Geometry check sheet. Reference: the model listing, model coordinates, mm. Face numbers are marked on the shaded views. A direction names the side the tool comes from. Give positions to 0.01 mm unless a question says otherwise; leave off trailing zeros. Loops run counter-clockwise (first coordinate to the right, second up) from the corner with the lowest first, then second, coordinate; pieces in that order, holes last.
1. Cross-section at A-A, the plane x = 0. Record the cut outline in (y, z), plus the area to 3 significant figures.
2. Release check for a two-part mould opening along Y. For the marked faces 4, 5 and 6 record: +Y half, -Y half, draft (parallel to the pull), parting line (faces both ways), or undercut.
3. Cross-section at D-D, the plane x = 6.5. Record the cut outline in (y, z), plus the area to 3 significant figures.
4. Cross-section at B-B, the plane z = 0. Record the cut outline in (x, y).
5. Cross-section at C-C, the plane y = -9.25. Record the cut outline in (x, z), plus the area to 3 significant figures.
6. Go/stop test with flat-tipped pins: pin 1 Ø7 at (x, z) = (0, 1.5) entering from +Y; pin 2 Ø8 at (x, y) = (8.5, 0.5) entering from -Z; pin 3 Ø1.5 at (x, y) = (-3.5, -0.5) entering from +Z; pin 4 Ø1.9 at (x, z) = (-1, 0.5) entering from -Y. Record where each tip stops, or that it passes through.
7. Tool access check on the marked faces 1, 2 and 3. Record the directions out of +Z, -Z, +X, -X, +Y, -Y that give a thin tool (end or side, any length) a straight path to the whole face; none if there is none.
8. Material ranges on L1, parallel to Y at x = -9.5, z = 5; L2, parallel to X at y = 5.25, z = 0; L3, parallel to X at y = 10.1, z = 0, recorded low to high.
from build123d import *

# Parameters (mm, degrees)
SKETCH_1_R          = 11
EXTRUDE_3_DEPTH     = 11
SKETCH_1_10_R       = 11
SKETCH_1_10_R_2     = 5.5
CUT_EXTRUDE_1_DEPTH = 8
SKETCH_2_R          = 2
CUT_EXTRUDE_2_DEPTH = 27.944387171
SKETCH_2_3_R        = 3.1
CUT_EXTRUDE_3_DEPTH = 2.7
CUT_EXTRUDE_START   = -19.3
SKETCH_2_4_R        = 3.1
CUT_EXTRUDE_4_DEPTH = 2.7


with BuildPart() as part:
    # 草图1 → 凸台-拉伸3 (new, symmetric)
    with BuildSketch(Plane(origin=(0, 0, 0), x_dir=(1, 0, 0), z_dir=(0, 1, 0))):
        with Locations(Location((0, 0, 0), (0, 0, 270))):
            Circle(SKETCH_1_R)
    extrude(amount=EXTRUDE_3_DEPTH, both=True)

    # 草图1<10> → 切除-拉伸1 (cut, symmetric)
    with BuildSketch(Plane(origin=(0, 0, 0), x_dir=(1, 0, 0), z_dir=(0, 1, 0))):
        with Locations(Location((0, 0, 0), (0, 0, 270))):
            Circle(SKETCH_1_10_R)
        with Locations(Location((0, 0, 0), (0, 0, 270))):
            Circle(SKETCH_1_10_R_2, mode=Mode.SUBTRACT)
    extrude(amount=CUT_EXTRUDE_1_DEPTH, both=True, mode=Mode.SUBTRACT)

    # 草图2 → 切除-拉伸2 (cut, through all)
    with BuildSketch(Plane(origin=(0, 11, 0), x_dir=(1, 0, 0), z_dir=(0, 1, 0))):
        with Locations(Location((0, 0, 0), (0, 0, 270))):
            Circle(SKETCH_2_R)
    extrude(amount=-CUT_EXTRUDE_2_DEPTH, mode=Mode.SUBTRACT)

    # 草图2<3> → 切除-拉伸3 (cut)
    with BuildSketch(Plane(origin=(0, 11, 0), x_dir=(1, 0, 0), z_dir=(0, 1, 0))):
        with Locations(Location((0, 0, 0), (0, 0, 270))):
            Circle(SKETCH_2_3_R)
    extrude(amount=-CUT_EXTRUDE_3_DEPTH, mode=Mode.SUBTRACT)

    # 草图2<4> → 切除-拉伸4 (cut)
    with BuildSketch(Plane(origin=(0, 11, 0), x_dir=(1, 0, 0), z_dir=(0, 1, 0)).offset(CUT_EXTRUDE_START)):
        with Locations(Location((0, 0, 0), (0, 0, 270))):
            Circle(SKETCH_2_4_R)
    extrude(amount=-CUT_EXTRUDE_4_DEPTH, mode=Mode.SUBTRACT)


solid = part.part
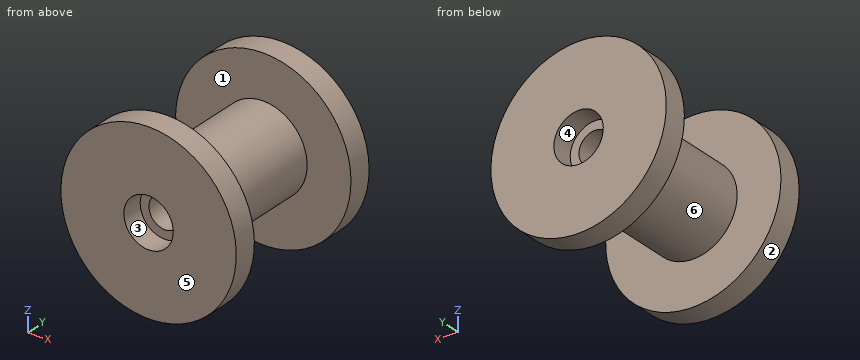
Result:
1. outline: (-11, -11) - (-8, -11) - (-8, -5.5) - (8, -5.5) - (8, -11) - (11, -11) - (11, -3.1) - (8.3, -3.1) - (8.3, -2) - (-8.3, -2) - (-8.3, -3.1) - (-11, -3.1) - close; (-11, 3.1) - (-8.3, 3.1) - (-8.3, 2) - (8.3, 2) - (8.3, 3.1) - (11, 3.1) - (11, 11) - (8, 11) - (8, 5.5) - (-8, 5.5) - (-8, 11) - (-11, 11) - close
1. area: 208 mm2
2. face 4: draft
2. face 5: -Y half
2. face 6: undercut
3. outline: (-11, -8.87) - (-8, -8.87) - (-8, 8.87) - (-11, 8.87) - close; (8, -8.87) - (11, -8.87) - (11, 8.87) - (8, 8.87) - close
3. area: 106 mm2
4. outline: (-11, -11) - (-3.1, -11) - (-3.1, -8.3) - (-2, -8.3) - (-2, 8.3) - (-3.1, 8.3) - (-3.1, 11) - (-11, 11) - (-11, 8) - (-5.5, 8) - (-5.5, -8) - (-11, -8) - close; (2, -8.3) - (3.1, -8.3) - (3.1, -11) - (11, -11) - (11, -8) - (5.5, -8) - (5.5, 8) - (11, 8) - (11, 11) - (3.1, 11) - (3.1, 8.3) - (2, 8.3) - close
5. outline: circle Ø22 at (0, 0); hole circle Ø6.2 at (0, 0)
5. area: 350 mm2
6. pin 1: stops at y = 11
6. pin 2: stops at z = -3.16
6. pin 3: stops at z = 4.76
6. pin 4: stops at y = -8.3
7. face 1: none
7. face 2: +Y, -Y
7. face 3: -Y
8. L1: y = -11 to -8, 8 to 11
8. L2: x = -5.5 to -2, 2 to 5.5
8. L3: x = -11 to -3.1, 3.1 to 11
